Autodesk Inventor part; units mm, degrees
ref_plane "YZ Plane" through (0, 0, 0) normal (1, 0, 0) x (0, 1, 0)
ref_plane "XZ Plane" through (0, 0, 0) normal (0, 1, 0) x (-1, 0, 0)
ref_plane "XY Plane" through (0, 0, 0) normal (0, 0, 1) x (1, 0, 0)
sketch "草图19" plane through (0, 0, 0) normal (0, 1, 0) x (-1, 0, 0)
  line L0 (-80, 80) -> (80, 80)
  line L1 (80, 80) -> (80, -80)
  line L2 (80, -80) -> (-80, -80)
  line L3 (-80, -80) -> (-80, 80)
  point P0 (0, 0)
  dimension "d55" = 160
  dimension "d56" = 160
extrude "拉伸19" add sketch "草图19" along normal blind 5
sketch "草图20" plane through (0, 5, 0) normal (0, 1, 0) x (1, 0, 0)
  circle A0 centre (15, -69) radius 1.8
  point P0 (0, 0)
  dimension "d59" = 3.6
extrude "拉伸20" cut sketch "草图20" against normal through all
sketch "草图21" plane through (0, 0, 0) normal (0, -1, 0) x (1, 0, 0)
  circle A0 centre (-15, 69) radius 1.8
  point P0 (0, 0)
  dimension "d62" = 3.6
extrude "拉伸21" cut sketch "草图21" against normal through all
sketch "草图26" plane through (0, 0, 0) normal (0, -1, 0) x (1, 0, 0)
  circle A0 centre (15, 45) radius 1.8
  point P0 (0, 0)
  dimension "d73" = 3.6
extrude "拉伸24" cut sketch "草图26" against normal through all
sketch "草图27" plane through (0, 0, 0) normal (0, -1, 0) x (1, 0, 0)
  circle A0 centre (-15, 45) radius 1.8
  point P0 (0, 0)
  dimension "d76" = 3.6
extrude "拉伸25" cut sketch "草图27" against normal through all
sketch "草图28" plane through (0, 0, 0) normal (0, -1, 0) x (1, 0, 0)
  circle A0 centre (45, 15) radius 1.8
  point P0 (0, 0)
  dimension "d79" = 3.6
extrude "拉伸26" cut sketch "草图28" against normal through all
sketch "草图29" plane through (0, 0, 0) normal (0, -1, 0) x (1, 0, 0)
  circle A0 centre (45, -15) radius 1.8
  point P0 (0, 0)
  dimension "d82" = 3.6
extrude "拉伸27" cut sketch "草图29" against normal through all
sketch "草图30" plane through (0, 0, 0) normal (0, -1, 0) x (1, 0, 0)
  circle A0 centre (69, 15) radius 1.8
  point P0 (0, 0)
  dimension "d85" = 3.6
extrude "拉伸28" cut sketch "草图30" against normal through all
sketch "草图31" plane through (0, 0, 0) normal (0, -1, 0) x (1, 0, 0)
  circle A0 centre (69, -15) radius 1.8
  point P0 (0, 0)
  dimension "d88" = 3.6
extrude "拉伸29" cut sketch "草图31" against normal through all
sketch "草图32" plane through (0, 0, 0) normal (0, -1, 0) x (1, 0, 0)
  circle A0 centre (-69, 15) radius 1.8
  point P0 (0, 0)
  dimension "d91" = 3.6
extrude "拉伸30" cut sketch "草图32" against normal through all
sketch "草图33" plane through (0, 0, 0) normal (0, -1, 0) x (1, 0, 0)
  circle A0 centre (-45, 15) radius 1.8
  point P0 (0, 0)
  dimension "d94" = 3.6
extrude "拉伸31" cut sketch "草图33" against normal through all
sketch "草图34" plane through (0, 0, 0) normal (0, -1, 0) x (1, 0, 0)
  circle A0 centre (-69, -15) radius 1.8
  point P0 (0, 0)
  dimension "d97" = 3.6
extrude "拉伸32" cut sketch "草图34" against normal through all
sketch "草图35" plane through (0, 0, 0) normal (0, -1, 0) x (1, 0, 0)
  circle A0 centre (-45, -15) radius 1.8
  point P0 (0, 0)
  dimension "d100" = 3.6
extrude "拉伸33" cut sketch "草图35" against normal through all
sketch "草图36" plane through (0, 0, 0) normal (0, -1, 0) x (1, 0, 0)
  point P0 (0, 0)
sketch "草图37" plane through (0, 0, 0) normal (0, -1, 0) x (1, 0, 0)
  circle A0 centre (0, -46) radius 3
  point P0 (0, 0)
  dimension "d103" = 6
extrude "拉伸34" cut sketch "草图37" against normal through all
sketch "草图38" plane through (0, 0, 0) normal (0, -1, 0) x (1, 0, 0)
  circle A0 centre (-16, -46) radius 2.5
  point P0 (0, 0)
  dimension "d106" = 5
extrude "拉伸35" cut sketch "草图38" against normal through all
sketch "草图39" plane through (0, 0, 0) normal (0, -1, 0) x (1, 0, 0)
  circle A0 centre (16, -46) radius 2.5
  point P0 (0, 0)
  dimension "d109" = 5
extrude "拉伸36" cut sketch "草图39" against normal through all
sketch "草图40" plane through (0, 0, 0) normal (0, -1, 0) x (1, 0, 0)
  circle A0 centre (-16, -76) radius 2.5
  point P0 (0, 0)
  dimension "d112" = 5
extrude "拉伸37" cut sketch "草图40" against normal through all
sketch "草图41" plane through (0, 0, 0) normal (0, -1, 0) x (1, 0, 0)
  circle A0 centre (16, -76) radius 2.5
  point P0 (0, 0)
  dimension "d115" = 5
extrude "拉伸38" cut sketch "草图41" against normal through all
sketch "草图42" plane through (0, 0, 0) normal (0, -1, 0) x (1, 0, 0)
  point P0 (0, 0)
equation "\"折弯半径\" = 厚度"
equation "\"折弯释压宽度\" = 厚度"
equation "\"折弯释压深度\" = 0.5 * 厚度"
equation "\"拐角释压尺寸\" = 4 * 厚度"
equation "\"最小余量\" = 2 * 厚度"
equation "\"过渡半径\" = 折弯半径"
equation "\"Jacobi半径尺寸\" = 折弯半径"
equation "\"间隙大小\" = 厚度"
properties part number "内层板"
Design review of the part built by this model. Coordinates are the model's own, in mm. Round coordinates to 2 decimals unless told otherwise and drop trailing zeros. Write each loop counter-clockwise with the first axis right and the second up, starting at its lowest first coordinate (ties: lowest second). Pieces come first, ordered by that corner, then holes. Notation, with made-up numbers: (80, 29.5) -> (96, 29.5) arc R18 ccw to (96, 57.5) -> close; hole circle Ø8 at (64.25, -3). An arc over 180 degrees is marked (long way). One line per question, with ' | ' between items.
(1) Insertion check: P1, Ø3, axis at x = -69, z = 15, coming from the +Y side; P2, Ø6, axis at x = 6, z = -33.5, coming from the -Y side. Each pin has a flat end and moves straight along its axis. Give the tip position at first contact, or say it passes through.
Result sheet:
P1: through | P2: y = 0
(2) Take a section at A-A, the plane z = -46. State the section outline as (x, y) points, and give its area (3 significant figures).
Result sheet:
outline: (-80, 0) -> (-18.5, 0) -> (-18.5, 5) -> (-80, 5) -> close; (-13.5, 0) -> (-3, 0) -> (-3, 5) -> (-13.5, 5) -> close; (3, 0) -> (13.5, 0) -> (13.5, 5) -> (3, 5) -> close; (18.5, 0) -> (80, 0) -> (80, 5) -> (18.5, 5) -> close | area: 720 mm2
(3) Take a section at C-C, the plane x = 0. State the section outline as (y, z) points.
Result sheet:
outline: (0, -80) -> (5, -80) -> (5, -49) -> (0, -49) -> close; (0, -43) -> (5, -43) -> (5, 80) -> (0, 80) -> close
(4) Wall thickness on line 1 (Z direction, x = 45, y = 2); line 2 (X direction, y = 2.3, z = 15.5); line 3 (Z direction, x = 2.5, y = 1.4): over which ranges is each line inside the solid? List them lowest first. Write a range as [from, to].
Result sheet:
line 1: [-80, -16.8], [-13.2, 13.2], [16.8, 80] | line 2: [-80, -70.73], [-67.27, -46.73], [-43.27, 43.27], [46.73, 67.27], [70.73, 80] | line 3: [-80, -47.66], [-44.34, 80]
(5) Draft analysis for pull direction X (two halves, no side actions). For faces 1 (the flat face through (1, 0, 1)), 2 (the cylindrical face through (-44.032, 2.465, -13.482)), 3 (the flat face through (-80, 2, 1)), 4 (the cylindrical face through (-16.54, 2.46, -48.44)), state which applies: released by +X, released by -X, zero draft, split by the parting line, or undercut.
Result sheet:
face 1: zero draft | face 2: undercut | face 3: released by -X | face 4: undercut
(6) Take a section at B-B, the plane z = -76. State the section outline as (x, y) points, and give its area (3 significant figures).
Result sheet:
outline: (-80, 0) -> (-18.5, 0) -> (-18.5, 5) -> (-80, 5) -> close; (-13.5, 0) -> (13.5, 0) -> (13.5, 5) -> (-13.5, 5) -> close; (18.5, 0) -> (80, 0) -> (80, 5) -> (18.5, 5) -> close | area: 750 mm2
